The listing builds one solid part. Answer for the finished solid, in the listing's coordinates (mm). A direction names the side the tool comes from. Round coordinates to 2 decimals unless told otherwise and drop trailing zeros. Loops run counter-clockwise (first coordinate to the right, second up) from the corner with the lowest first, then second, coordinate; pieces in that order, holes last. Notation, with made-up numbers: (79.25, 34.5) - (102.25, 34.5) arc R14 ccw to (102.25, 46.5) - close; hole circle Ø5 at (9.5, 14.5). An arc over 180 degrees is marked (long way). One line per item, written item: value.
```python
from build123d import *

# Parameters (mm, degrees)
F1_DEPTH  = 60
F2_W      = 100
F2_H      = 100
F3_DEPTH  = 22
F5_DEPTH  = 11.1
F6_W      = 15
F6_H      = 8
F7_DEPTH  = 12
F8_W      = 6
F8_H      = 8
F9_DEPTH  = 60.001
F10_W     = 2
F10_H     = 3
F10_H_2   = 4
F11_DEPTH = 60.001
F12_W     = 30
F12_H     = 15
F13_DEPTH = 22
F14_SIZE  = 3
F15_R     = 5
F16_SIZE  = 3.5


with BuildPart() as f1:
    # F0 (on Front) → F1 (new body)
    with BuildSketch(Plane.XZ):
        Polygon((0, 4), (0, 0), (25, 0), (25, 20), (46, 20), (46, 0), (56, 0), (56, 43), (41, 43), (41, 23), (10, 23), (10, 4), align=None)
    extrude(amount=-F1_DEPTH)

    # F2 (on face) → F3 (cut)
    with BuildSketch(Plane(origin=(0, 60, 0), x_dir=(-1, 0, 0), z_dir=(0, 1, 0))):
        with Locations((-50, 54)):
            Rectangle(F2_W, F2_H)
    extrude(amount=-F3_DEPTH, mode=Mode.SUBTRACT)

    # F4 (on face) → F5 (cut)
    with BuildSketch(Plane(origin=(0, 38, 0), x_dir=(-1, 0, 0), z_dir=(0, 1, 0))):
        Polygon((-110, 23), (-41, 23), (-10, 23), (-10, 123), (-110, 123), align=None)
    extrude(amount=-F5_DEPTH, mode=Mode.SUBTRACT)

    # F6 (on Front) → F7 (cut)
    with BuildSketch(Plane.XZ):
        with Locations((48.5, 33)):
            Rectangle(F6_W, F6_H)
    extrude(amount=-F7_DEPTH, mode=Mode.SUBTRACT)

    # F8 (on Front) → F9 (cut, through all)
    with BuildSketch(Plane.XZ):
        with Locations((53, 33)):
            Rectangle(F8_W, F8_H)
    extrude(amount=-F9_DEPTH, mode=Mode.SUBTRACT)

    # F10 (on Front) → F11 (cut, through all)
    with BuildSketch(Plane.XZ):
        with Locations((11, 5.5)):
            Rectangle(F10_W, F10_H)
        with Locations((11, 21)):
            Rectangle(F10_W, F10_H_2)
    extrude(amount=-F11_DEPTH, mode=Mode.SUBTRACT)

    # F12 (on face) → F13 (cut, through all)
    with BuildSketch(Plane(origin=(0, 60, 0), x_dir=(-1, 0, 0), z_dir=(0, 1, 0))):
        with Locations((-45, 7.5)):
            Rectangle(F12_W, F12_H)
    extrude(amount=-F13_DEPTH, mode=Mode.SUBTRACT)

    # F14
    f14_edges = [f1.edges().sort_by_distance(p)[0] for p in [
        (56, 19, 0),
        (0, 30, 0),
    ]]
    chamfer(f14_edges, length=F14_SIZE)

    # F15
    f15_edges = [f1.edges().sort_by_distance(p)[0] for p in [
        (50, 12, 33),
    ]]
    fillet(f15_edges, radius=F15_R)

    # F16
    f16_edges = [f1.edges().sort_by_distance(p)[0] for p in [
        (43, 12, 37),
        (43, 12, 29),
    ]]
    chamfer(f16_edges, length=F16_SIZE)


solid = f1.part
```
1) A cutting plane is placed at D-D on z = 36. Give the vertices of the cut face in (x, y), and give its area (3 significant figures).
Final values:
outline: (41, 9.5) - (45, 9.5) arc R7.5 ccw to (52.5, 17) - (52.5, 26.9) - (41, 26.9) - close
area: 188 mm2
2) Each of these flat-tipped pins is pushed along its axis until it touches: pin 1 Ø10 at (y, z) = (9.5, 29) entering from -X; pin 2 Ø12 at (x, z) = (47, 35) entering from +Y; pin 3 Ø7.5 at (x, y) = (16, 39.5) entering from +Z. Where does it stop, or does it pass through?
Final values:
pin 1: x = 41
pin 2: y = 26.9
pin 3: z = 23
3) A cutting plane is placed at B-B on y = 34. Give the vertices of the cut face in (x, z), and give its area (3 significant figures).
Final values:
outline: (0, 3) - (3, 0) - (25, 0) - (25, 20) - (46, 20) - (46, 0) - (53, 0) - (56, 3) - (56, 23) - (12, 23) - (12, 19) - (10, 19) - (10, 7) - (12, 7) - (12, 4) - (0, 4) - close
area: 655 mm2
4) A cutting plane is placed at C-C on x = 23.5. Give the vertices of the cut face in (y, z), and give its area (3 significant figures).
Final values:
outline: (0, 0) - (60, 0) - (60, 4) - (38, 4) - (38, 23) - (0, 23) - close
area: 962 mm2
5) Consider L1, parallel to X at y = 12, z = 13.5; L2, parallel to X at y = 23, z = 5; L3, parallel to Z at x = 28, y = 7. Determine where each line is inside the solid, lowest interval first.
Final values:
L1: 10 to 25, 46 to 56
L2: 12 to 25, 46 to 56
L3: 20 to 23
6) For a pull along X with two mould halves and no side action, classify faces 5 (the conical face through (49.431, 12.47, 31.163)), 6 (the flat face through (35, 19, 20)), 7 (the flat face through (11, 19, 19)) as released by +X, released by -X, zero draft, split by the parting line, or undercut.
Final values:
face 5: released by +X
face 6: undercut
face 7: zero draft
7) A cutting plane is placed at A-A on z = 11. Give the vertices of the cut face in (x, y).
Final values:
outline: (10, 0) - (25, 0) - (25, 38) - (10, 38) - close; (46, 0) - (56, 0) - (56, 38) - (46, 38) - close
8) For faces 1 (the flat face through (49, 26.9, 33)), 2 (the flat face through (12, 19, 5)), 3 (the flat face through (46, 19, 10)), 4 (the conical face through (49.465, 12.435, 34.886)), determine the directions among +Z, -Z, +X, -X, +Y, -Y from which every point of the face is accessible in a straight line to the end or side of a thin tool.
Final values:
face 1: +Z, +X, -X, +Y
face 2: -X, +Y, -Y
face 3: -Z, +Y, -Y
face 4: +X, -Y
